For this review, take the finished solid that the model builds, in its own axes (mm). A direction names the side the tool comes from. Round coordinates to 2 decimals unless told otherwise and drop trailing zeros. Write each loop counter-clockwise with the first axis right and the second up, starting at its lowest first coordinate (ties: lowest second). Pieces come first, ordered by that corner, then holes.
from build123d import *

# Parameters (mm, degrees)
F1_DEPTH = 25.4
F2_R     = 6.35
F3_R     = 7.9375
F4_DEPTH = 25.401


with BuildPart() as f1:
    # F0 (on Top) → F1 (new body)
    with BuildSketch(Plane.XY):
        with BuildLine():
            Line((0, 9.201151), (0, 0))
            Line((0, 0), (139.7, 0))
            Line((139.7, 0), (139.7, 12.7))
            Line((139.7, 12.7), (226.906916, 12.7))
            ThreePointArc((226.906916, 12.7), (265.176, 31.75), (226.906916, 50.8))
            Line((226.906916, 50.8), (139.7, 50.8))
            Line((139.7, 50.8), (139.7, 63.5))
            Line((139.7, 63.5), (0, 63.5))
            Line((0, 63.5), (0, 54.298849))
            ThreePointArc((0, 54.298849), (9.398, 31.75), (0, 9.201151))
        make_face()
    extrude(amount=F1_DEPTH)

    # F2
    f2_edges = [f1.edges().sort_by_distance(p)[0] for p in [
        (139.7, 0, 12.7),
        (139.7, 63.5, 12.7),
        (226.906916, 12.7, 12.7),
        (226.906916, 50.8, 12.7),
    ]]
    fillet(f2_edges, radius=F2_R)

    # F3 (on face) → F4 (cut, through all)
    with BuildSketch(Plane.XY.offset(25.4)):
        with Locations((241.3, 31.75)):
            Circle(F3_R)
    extrude(amount=-F4_DEPTH, mode=Mode.SUBTRACT)


solid = f1.part
(1) Mouldability with a two-part tool opening along Y and no side actions: class faces 4 (the face through (137.79, 1.81, 12.88)), 5 (the face through (233.37, 32.1, 12.88)), 6 (the face through (9.396, 32.101, 12.522)), 7 (the face through (183, 50.8, 13)) as pulls with the +Y half, pulls with the -Y half, needs draft (parallel to the pull), parting line crosses it, or undercut.
Geometry check:
face 4: pulls with the -Y half
face 5: undercut
face 6: undercut
face 7: pulls with the +Y half
(2) For faces 1 (the face through (265.165, 31.034, 12.522)), 2 (the face through (139.7, 9, 13)), 3 (the face through (139.7, 54, 13)), list the 3-axis set-ups (+Z, -Z, +X, -X, +Y, -Y) from which the entire face can be reached by the end or side of a thin tool; tool diameter is ignored.
Geometry check:
face 1: +Z, -Z
face 2: +Z, -Z, -Y
face 3: +Z, -Z, +Y
(3) We need section C-C, the plane x = 241.3. Give the boundary of the cut face in (y, z), and give its area (3 significant figures).
Geometry check:
outline: (7.87, 0) - (23.81, 0) - (23.81, 25.4) - (7.87, 25.4) - close; (39.69, 0) - (55.63, 0) - (55.63, 25.4) - (39.69, 25.4) - close
area: 810 mm2
(4) For pin 1 Ø10 at (x, y) = (43, 27.5) entering from -Z; pin 2 Ø10 at (y, z) = (45, 11.5) entering from -X; pin 3 Ø5 at (y, z) = (11, 11) entering from +X; pin 4 Ø1.9 at (y, z) = (54.5, 18.5) entering from +X, all flat-tipped, find the tip position at first contact; note any pin that passes through.
Geometry check:
pin 1: stops at z = 0
pin 2: stops at x = 3.63
pin 3: stops at x = 256.69
pin 4: stops at x = 251.04
(5) For line 1 along Y through (x, z) = (241.3, 18); line 2 along Y through (x, z) = (206, 12.5); line 3 along Y through (x, z) = (243, 19.25), list the stretches that pass through material, from the lowest coordinate up.
Geometry check:
line 1: y = 7.87 to 23.81, 39.69 to 55.63
line 2: y = 12.7 to 50.8
line 3: y = 7.93 to 24, 39.5 to 55.57
(6) We need section A-A, the plane y = 31.75. Give the boundary of the cut face in (x, z).
Geometry check:
outline: (9.4, 0) - (233.36, 0) - (233.36, 25.4) - (9.4, 25.4) - close; (249.24, 0) - (265.18, 0) - (265.18, 25.4) - (249.24, 25.4) - close
(7) We need section D-D, the plane x = 168. Give the boundary of the cut face in (y, z).
Geometry check:
outline: (12.7, 0) - (50.8, 0) - (50.8, 25.4) - (12.7, 25.4) - close
